Study the drawing (mm; zero at the part's minimum x, y, z) and answer. A direction names the side the tool comes from. Coordinates: 2 decimals unless noted, no trailing zeros. Order: outer loops, then holes, each group sorted by start corner. A loop starts at its lowest first (then second) coordinate and runs counter-clockwise, first axis right, second up.
1. Flat-ended cylindrical pins translate along their axes: pin 1 Ø1.8 at (y, z) = (40.5, 36.5) entering from -X; pin 2 Ø1 at (y, z) = (13, 12.5) entering from -X; pin 3 Ø12.5 at (x, z) = (28, 28) entering from -Y. Find the tip coordinate at first contact, or state that the pin passes through.
2. The part is cut by section D-D, the plane y = 23.5. Give the vertices of the cut face in (x, z), then the cut area to 3 significant figures.
3. The part is cut by section A-A, the plane x = 14.5. Give the vertices of the cut face in (y, z).
4. A tool of negligible diameter and unlimited length cuts with its end or side. For the marked faces 1 and 2, from which of +Z, -Z, +X, -X, +Y, -Y can it reach the whole face along a straight path? Write none if from no direction.
5. Find the intervals of material crossed by probe 1 along Y at (x, z) = (42.9, 36.5); probe 2 along Y at (x, z) = (42.9, 21); probe 3 along Y at (x, z) = (43, 36), in increasing order.
6. The part is cut by section C-C, the plane z = 5.5. Give the vertices of the cut face in (x, y), then the cut area to 3 significant figures.
7. The part is cut by section B-B, the plane y = 9.5. Give the vertices of the cut face in (x, z), then the cut area to 3 significant figures.
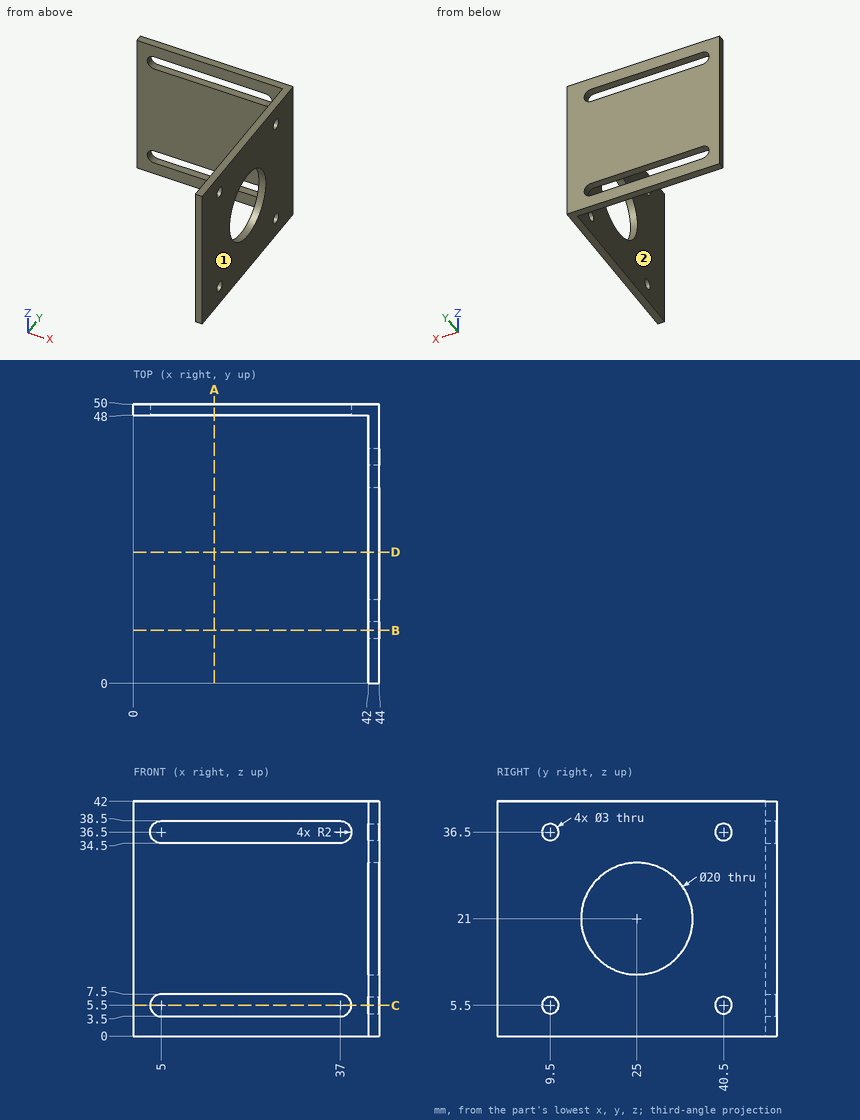
Geometry says:
1. pin 1: passes through
1. pin 2: stops at x = 42
1. pin 3: stops at y = 48
2. outline: (42, 0) - (44, 0) - (44, 11.11) - (42, 11.11) - close; (42, 30.89) - (44, 30.89) - (44, 42) - (42, 42) - close
2. area: 44.5 mm2
3. outline: (48, 0) - (50, 0) - (50, 3.5) - (48, 3.5) - close; (48, 7.5) - (50, 7.5) - (50, 34.5) - (48, 34.5) - close; (48, 38.5) - (50, 38.5) - (50, 42) - (48, 42) - close
4. face 1: +Z, -Z, +X, +Y, -Y
4. face 2: +Z, -Z, -X, -Y
5. probe 1: y = 0 to 8, 11 to 39, 42 to 50
5. probe 2: y = 0 to 15, 35 to 50
5. probe 3: y = 0 to 8.09, 10.91 to 39.09, 41.91 to 50
6. outline: (0, 48) - (3, 48) - (3, 50) - (0, 50) - close; (39, 48) - (42, 48) - (42, 42) - (44, 42) - (44, 50) - (39, 50) - close; (42, 0) - (44, 0) - (44, 8) - (42, 8) - close; (42, 11) - (44, 11) - (44, 39) - (42, 39) - close
6. area: 100 mm2
7. outline: (42, 0) - (44, 0) - (44, 4) - (42, 4) - close; (42, 7) - (44, 7) - (44, 35) - (42, 35) - close; (42, 38) - (44, 38) - (44, 42) - (42, 42) - close
7. area: 72.0 mm2
